Study the drawing (mm; zero at the part's minimum x, y, z) and answer. Give positions to 0.01 mm unless a question says otherwise; leave off trailing zeros. Order: outer loops, then holes, each group sorted by start corner. A loop starts at its lowest first (then second) coordinate and runs counter-clockwise, first axis right, second up.
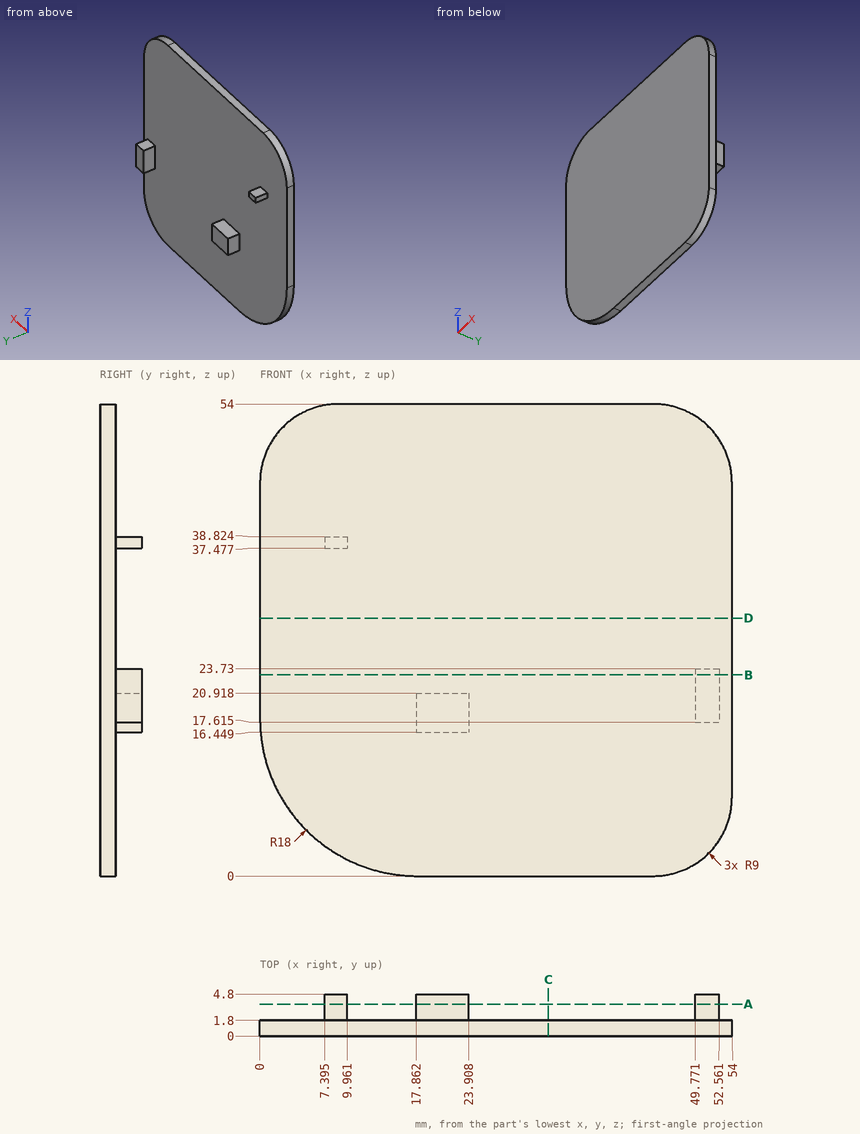
1) Find section C-C (x = 33). Write down the section's boundary in (y, z).
Geometry says:
outline: (0, 0) - (1.8, 0) - (1.8, 54) - (0, 54) - close
2) Given P1, Ø12, axis at x = 32, z = 45.5, coming from the +Y side; P2, Ø0.8, axis at x = 51, y = 3.5, coming from the -Z side (1 decimal); P3, Ø1.5, axis at x = 19.5, y = 4, coming from the +Z side, each flat-ended and moving along its own axis, determine where each tip first touches the part or whether it passes through.
Geometry says:
P1: stops at y = 1.8
P2: stops at z = 17.6
P3: stops at z = 20.92
3) Find section A-A (y = 3.65). Write down the section's boundary in (x, z) (1 decimal).
Geometry says:
outline: (7.4, 37.5) - (10, 37.5) - (10, 38.8) - (7.4, 38.8) - close; (17.9, 16.4) - (23.9, 16.4) - (23.9, 20.9) - (17.9, 20.9) - close; (49.8, 17.6) - (52.6, 17.6) - (52.6, 23.7) - (49.8, 23.7) - close
4) Straight lines are drawn through the part: probe 1 along Y at (x, z) = (34, 11); probe 2 along X at (y, z) = (3.65, 19); probe 3 along Z at (x, y) = (51, 4.25) (1 decimal). For each, find the intervals that lie inside material, in ascending order.
Geometry says:
probe 1: y = 0 to 1.8
probe 2: x = 17.86 to 23.91, 49.77 to 52.56
probe 3: z = 17.6 to 23.7
5) Find section B-B (z = 23). Write down the section's boundary in (x, y).
Geometry says:
outline: (0, 0) - (54, 0) - (54, 1.8) - (52.56, 1.8) - (52.56, 4.8) - (49.77, 4.8) - (49.77, 1.8) - (0, 1.8) - close
6) Find section D-D (z = 29.5). Write down the section's boundary in (x, y).
Geometry says:
outline: (0, 0) - (54, 0) - (54, 1.8) - (0, 1.8) - close
